The model under review builds one solid part; all positions refer to its coordinate system, in mm. A direction names the side the tool comes from. Give positions to 0.01 mm unless a question says otherwise; leave off trailing zeros. Order: outer loops, then holes, each group sorted by start corner. A loop starts at its lowest first (then second) coordinate and runs counter-clockwise, first axis right, second up. Notation, with made-up numbers: (-1, 32) - (36, 32) arc R20 ccw to (36, 67) - close; hole circle Ø4 at (80.25, 51). An arc over 180 degrees is marked (long way). Answer as CSV lines item,"result". Start each with the question number.
from build123d import *

# Parameters (mm, degrees)
F0_W         = 9.9060004577
F0_H         = 18.2879995555
F1_DEPTH     = 6.35
F2_W         = 9.9060004577
F2_H         = 18.2879995555
F3_DEPTH     = 15.24
F4_T1_DEPTH  = 140.9700014576
F4_T3_DEPTH  = 65.5320005
F4_T5_DEPTH  = 65.5320005
F4_T10_DEPTH = 140.9700014576
F4_T16_DEPTH = 140.9700014576
F4_T22_DEPTH = 140.9700014576
F4_T29_DEPTH = 140.9700014576
F4_T35_DEPTH = 140.9700014576
F4_T41_DEPTH = 84.5820005
F4_T46_DEPTH = 84.5820005


# Not quite as in the source:
# - a fillet or chamfer that OpenCascade refuses, or shapes differently, is made with other operations: its cross-section is extruded or revolved along the edge and cut away or added


with BuildPart() as f1:
    # F0 (on Front) → F1 (new body, symmetric)
    with BuildSketch(Plane.XZ):
        with Locations((-4.9530002289, 9.1439997777)):
            Rectangle(F0_W, F0_H)
    extrude(amount=F1_DEPTH, both=True)

    # F2 (on face) → F3 (join)
    with BuildSketch(Plane(origin=(0, 6.35, 0), x_dir=(-1, 0, 0), z_dir=(0, 1, 0))):
        Polygon((0, 18.2879995555), (-46.4820005, 18.2879995555), (-46.4820005, -0.6095990539), (56.3880009577, -0.6095990539), (56.3880009577, 18.2879995555), (9.9060004577, 18.2879995555), (9.9060004577, 0), (0, 0), align=None)
        with Locations((4.9530002289, 9.1439997777)):
            Rectangle(F2_W, F2_H)
    extrude(amount=F3_DEPTH)

    # F4: fillet of radius 7.62 on 5 edges, made by hand

    # F4_s2 → F4_t1 (cut)
    with BuildSketch(Plane.YZ.offset(-75.4380009577)):
        with BuildLine():
            ThreePointArc((13.97, -0.6095990539), (19.3581536726, 1.6222472735), (21.59, 7.0104009461))
            Line((21.59, 7.0104009461), (21.59, -0.6095990539))
            Line((21.59, -0.6095990539), (13.97, -0.6095990539))
        make_face()
        with BuildLine():
            ThreePointArc((13.97, 18.2879995555), (19.3581536726, 16.0561532281), (21.59, 10.6679995555))
            Line((21.59, 10.6679995555), (21.59, 18.2879995555))
            Line((21.59, 18.2879995555), (13.97, 18.2879995555))
        make_face()
    extrude(amount=F4_T1_DEPTH, mode=Mode.SUBTRACT)

    # F4_s4 → F4_t3 (cut)
    with BuildSketch(Plane.YZ.offset(-75.4380009577)):
        with BuildLine():
            ThreePointArc((13.97, 18.2879995555), (8.5818463274, 16.0561532281), (6.35, 10.6679995555))
            Line((6.35, 10.6679995555), (6.35, 18.2879995555))
            Line((6.35, 18.2879995555), (13.97, 18.2879995555))
        make_face()
    extrude(amount=F4_T3_DEPTH, mode=Mode.SUBTRACT)

    # F4_s6 → F4_t5 (cut)
    with BuildSketch(Plane.YZ):
        with BuildLine():
            ThreePointArc((13.97, 18.2879995555), (8.5818463274, 16.0561532281), (6.35, 10.6679995555))
            Line((6.35, 10.6679995555), (6.35, 18.2879995555))
            Line((6.35, 18.2879995555), (13.97, 18.2879995555))
        make_face()
    extrude(amount=F4_T5_DEPTH, mode=Mode.SUBTRACT)


with BuildPart() as f4_tool8:
    # F4_s9 → F4_t10 (new body)
    with BuildSketch(Plane.YZ.offset(65.5320005)):
        with BuildLine():
            ThreePointArc((13.97, -0.6095990539), (8.5818463274, 1.6222472735), (6.35, 7.0104009461))
            Line((6.35, 7.0104009461), (6.35, -0.6095990539))
            Line((6.35, -0.6095990539), (13.97, -0.6095990539))
        make_face()
    extrude(amount=-F4_T10_DEPTH)

    split(bisect_by=Plane.YZ, keep=Keep.TOP)

    split(bisect_by=Plane.XY, keep=Keep.BOTTOM)


with BuildPart() as f1_1:
    add(f1.part)

    # F4_t7: cut F4_tool8
    add(f4_tool8.part, mode=Mode.SUBTRACT)


with BuildPart() as f4_tool14:
    # F4_s15 → F4_t16 (new body)
    with BuildSketch(Plane.YZ.offset(65.5320005)):
        with BuildLine():
            ThreePointArc((13.97, -0.6095990539), (8.5818463274, 1.6222472735), (6.35, 7.0104009461))
            Line((6.35, 7.0104009461), (6.35, -0.6095990539))
            Line((6.35, -0.6095990539), (13.97, -0.6095990539))
        make_face()
    extrude(amount=-F4_T16_DEPTH)

    split(bisect_by=Plane.YZ, keep=Keep.TOP)

    split(bisect_by=Plane.XY, keep=Keep.TOP)


with BuildPart() as f1_2:
    add(f1_1.part)

    # F4_t13: cut F4_tool14
    add(f4_tool14.part, mode=Mode.SUBTRACT)


with BuildPart() as f4_tool20:
    # F4_s21 → F4_t22 (new body)
    with BuildSketch(Plane.YZ.offset(65.5320005)):
        with BuildLine():
            ThreePointArc((13.97, -0.6095990539), (8.5818463274, 1.6222472735), (6.35, 7.0104009461))
            Line((6.35, 7.0104009461), (6.35, -0.6095990539))
            Line((6.35, -0.6095990539), (13.97, -0.6095990539))
        make_face()
    extrude(amount=-F4_T22_DEPTH)

    split(bisect_by=Plane.YZ, keep=Keep.BOTTOM)

    split(bisect_by=Plane.XY, keep=Keep.BOTTOM)

    split(bisect_by=Plane.YZ.offset(-9.9060004577), keep=Keep.TOP)


with BuildPart() as f1_3:
    add(f1_2.part)

    # F4_t19: cut F4_tool20
    add(f4_tool20.part, mode=Mode.SUBTRACT)


with BuildPart() as f4_tool27:
    # F4_s28 → F4_t29 (new body)
    with BuildSketch(Plane.YZ.offset(65.5320005)):
        with BuildLine():
            ThreePointArc((13.97, -0.6095990539), (8.5818463274, 1.6222472735), (6.35, 7.0104009461))
            Line((6.35, 7.0104009461), (6.35, -0.6095990539))
            Line((6.35, -0.6095990539), (13.97, -0.6095990539))
        make_face()
    extrude(amount=-F4_T29_DEPTH)

    split(bisect_by=Plane.XY, keep=Keep.BOTTOM)

    split(bisect_by=Plane.YZ.offset(-9.9060004577), keep=Keep.BOTTOM)


with BuildPart() as f1_4:
    add(f1_3.part)

    # F4_t26: cut F4_tool27
    add(f4_tool27.part, mode=Mode.SUBTRACT)


with BuildPart() as f4_tool33:
    # F4_s34 → F4_t35 (new body)
    with BuildSketch(Plane.YZ.offset(65.5320005)):
        with BuildLine():
            ThreePointArc((13.97, -0.6095990539), (8.5818463274, 1.6222472735), (6.35, 7.0104009461))
            Line((6.35, 7.0104009461), (6.35, -0.6095990539))
            Line((6.35, -0.6095990539), (13.97, -0.6095990539))
        make_face()
    extrude(amount=-F4_T35_DEPTH)

    split(bisect_by=Plane.XY, keep=Keep.TOP)

    split(bisect_by=Plane.YZ.offset(-9.9060004577), keep=Keep.BOTTOM)


with BuildPart() as f1_5:
    add(f1_4.part)

    # F4_t32: cut F4_tool33
    add(f4_tool33.part, mode=Mode.SUBTRACT)


with BuildPart() as f4_tool39:
    # F4_s40 → F4_t41 (new body)
    with BuildSketch(Plane.YZ.offset(-75.4380009577)):
        with BuildLine():
            ThreePointArc((13.97, 18.2879995555), (8.5818463274, 16.0561532281), (6.35, 10.6679995555))
            Line((6.35, 10.6679995555), (6.35, 18.2879995555))
            Line((6.35, 18.2879995555), (13.97, 18.2879995555))
        make_face()
    extrude(amount=F4_T41_DEPTH)

    split(bisect_by=Plane.YZ, keep=Keep.TOP)


with BuildPart() as f1_6:
    add(f1_5.part)

    # F4_t38: cut F4_tool39
    add(f4_tool39.part, mode=Mode.SUBTRACT)


with BuildPart() as f4_tool44:
    # F4_s45 → F4_t46 (new body)
    with BuildSketch(Plane.YZ.offset(-19.05)):
        with BuildLine():
            ThreePointArc((13.97, 18.2879995555), (8.5818463274, 16.0561532281), (6.35, 10.6679995555))
            Line((6.35, 10.6679995555), (6.35, 18.2879995555))
            Line((6.35, 18.2879995555), (13.97, 18.2879995555))
        make_face()
    extrude(amount=F4_T46_DEPTH)

    split(bisect_by=Plane.YZ.offset(-9.9060004577), keep=Keep.BOTTOM)


with BuildPart() as f1_7:
    add(f1_6.part)

    # F4_t43: cut F4_tool44
    add(f4_tool44.part, mode=Mode.SUBTRACT)


solid = f1_7.part
Item 1: Machinability: for faces 1 (the face through (24, 6.35, 9)), 2 (the face through (-5, 2, 0)), 3 (the face through (-4.233, 14.138, -0.608)), 4 (the face through (-33, 6.35, 9)), which of the approach directions +Z, -Z, +X, -X, +Y, -Y give a long, thin tool a straight path to every point of the face, cutting with its end or side? Answer none if there is none.
Item 2: Take a section at A-A on z = 1.25. Write out the cut boundary in (x, y).
Item 3: For line 1 along X through (y, z) = (-2, 17.5); line 2 along Y through (x, z) = (-44.5, 10.5); line 3 along Z through (x, y) = (3, 13.5), list the stretches that pass through material, from the lowest coordinate up.
Item 4: Clearance check with flat-ended pins moving along their axes: pin 1 (9 mm diameter, centred on y = 4, z = 6.5, fed in from +X); pin 2 (1.5 mm diameter, centred on x = -12.5, z = 8.5, fed in from -Y); pin 3 (4 mm diameter, centred on x = -5, z = 3.5, fed in from +Y); pin 4 (2 mm diameter, centred on y = -1, z = 5.5, fed in from +X). State where each tip first meets the part, or that it passes through.
Item 5: Take a section at C-C on x = -3. Write out the cut boundary in (y, z), and give its area (3 significant figures).
Item 6: Take a section at B-B on y = 8.75. Write out the cut boundary in (x, z).
Item 7: Take a section at D-D on z = 17. Write out the cut boundary in (x, y).
Data:
1,face 1,"+Z, -Z, +X, -Y"
1,face 2,"-Z, +X, -X, -Y"
1,face 3,"-Z"
1,face 4,"+Z, -Z, -X, -Y"
2,outline,"(-56.39, 8.98) - (-9.91, 8.98) - (-9.91, -6.35) - (0, -6.35) - (0, 8.98) - (46.48, 8.98) - (46.48, 18.96) - (-56.39, 18.96) - close"
3,line 1,"x = -9.91 to 0"
3,line 2,"y = 6.35 to 21.59"
3,line 3,"z = -0.6 to 18.27"
4,pin 1,"stops at x = 46.48"
4,pin 2,"stops at y = 6.35"
4,pin 3,"stops at y = 21.44"
4,pin 4,"stops at x = 0"
5,outline,"(-6.35, 0) - (10.98, 0) arc R7.62 ccw to (21.59, 7.01) - (21.59, 10.67) arc R7.62 ccw to (13.97, 18.29) - (-6.35, 18.29) - close"
5,area,"492 mm^2"
6,outline,"(-56.39, 1.46) - (-9.91, 1.46) - (-9.91, 0) - (0, 0) - (0, 1.46) - (46.48, 1.46) - (46.48, 16.22) - (0, 16.22) - (0, 18.29) - (-9.91, 18.29) - (-9.91, 16.22) - (-56.39, 16.22) - close"
7,outline,"(-56.39, 9.73) - (-9.91, 9.73) - (-9.91, -6.35) - (0, -6.35) - (0, 9.73) - (46.48, 9.73) - (46.48, 18.21) - (-56.39, 18.21) - close"
